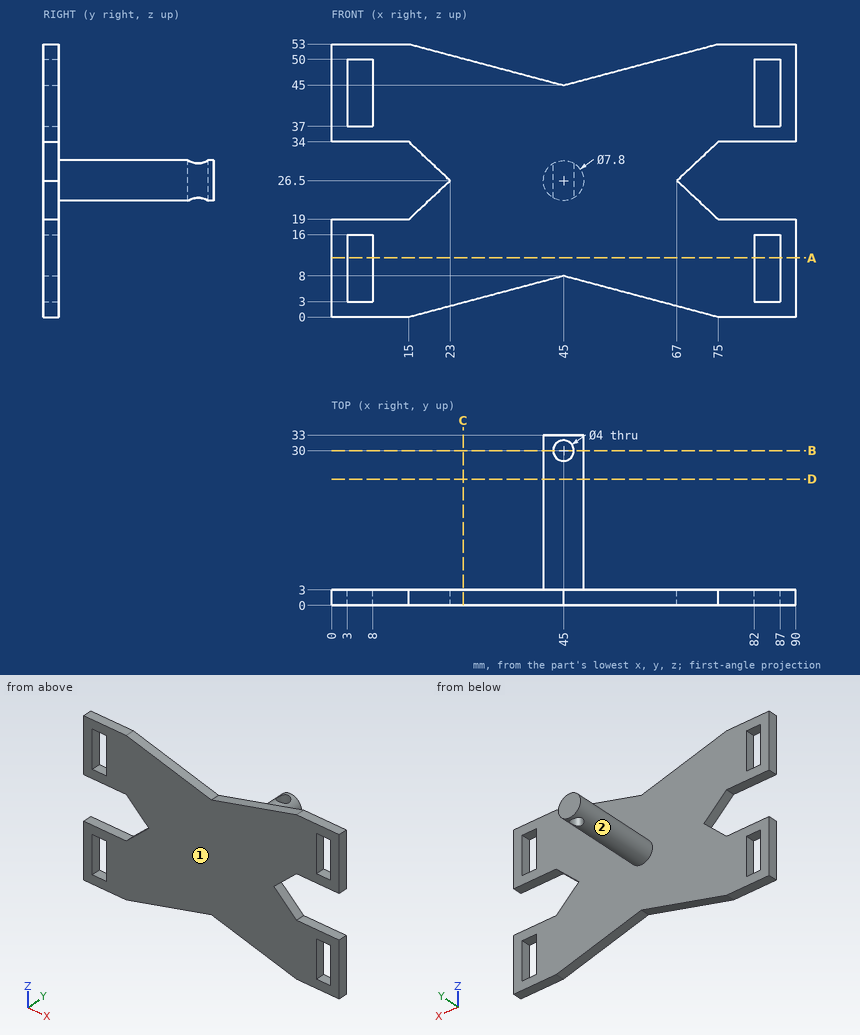
Answer from the drawing. Dimensions are ordinates in mm from the lowest x, y and z of the part. A direction names the side the tool comes from. Give positions to 0.01 mm unless a question says otherwise; leave off trailing zeros. Loops run counter-clockwise (first coordinate to the right, second up) from the corner with the lowest first, then second, coordinate; pieces in that order, holes last.
Item 1: The part is cut by section B-B (y = 30). Write down the section's boundary in (x, z), and give its area (3 significant figures).
Item 2: Each of these flat-tipped pins is pushed along its axis until it touches: pin 1 Ø1.5 at (x, y) = (80.5, 4) entering from -Z; pin 2 Ø4.5 at (x, y) = (45, 30) entering from +Z; pin 3 Ø16 at (x, z) = (63, 19.5) entering from +Y; pin 4 Ø6 at (y, z) = (26.5, 33) entering from +X. Where does it stop, or does it pass through?
Item 3: The part is cut by section D-D (y = 24.5). Write down the section's boundary in (x, z), and give its area (3 significant figures).
Item 4: The part is cut by section A-A (z = 11.5). Write down the section's boundary in (x, y), and give its area (3 significant figures).
Item 5: Find the intervals of material crossed by line 1 along Y through (x, z) = (45, 26); line 2 along Y through (x, z) = (24, 3); line 3 along X through (y, z) = (30, 27.75), in increasing order.
Item 6: The part is cut by section C-C (x = 25.5). Write down the section's boundary in (y, z), and give its area (3 significant figures).
Item 7: For the marked faces 1 and 2, determine the directions among +Z, -Z, +X, -X, +Y, -Y from which every point of the face is accessible in a straight line to the end or side of a thin tool.
Taken from the geometry:
1. outline: (43, 23.15) - (43, 29.85) arc R3.9 ccw to start; (47, 23.15) arc R3.9 ccw to (47, 29.85) - close
1. area: 18.0 mm2
2. pin 1: passes through
2. pin 2: stops at z = 30.4
2. pin 3: stops at y = 3
2. pin 4: stops at x = 46.72
3. outline: circle Ø7.8 at (45, 26.5)
3. area: 47.8 mm2
4. outline: (0, 0) - (3, 0) - (3, 3) - (0, 3) - close; (8, 0) - (82, 0) - (82, 3) - (8, 3) - close; (87, 0) - (90, 0) - (90, 3) - (87, 3) - close
4. area: 240 mm2
5. line 1: y = 0 to 28, 32 to 33
5. line 2: y = 0 to 3
5. line 3: x = 41.31 to 43, 47 to 48.69
6. outline: (0, 2.8) - (3, 2.8) - (3, 50.2) - (0, 50.2) - close
6. area: 142 mm2
7. face 1: +Z, -Z, +X, -X, -Y
7. face 2: +Y
